Read the model definition and answer for the solid it produces. Units are mm, in the model's axes. Face numbers are marked on the shaded views. Coordinates: 2 decimals unless noted, no trailing zeros. Write each loop counter-clockwise with the first axis right and the second up, starting at its lowest first coordinate (ties: lowest second). Pieces come first, ordered by that corner, then holes. Notation, with made-up numbers: (-14.75, 50.5) -> (4.25, 50.5) arc R20 ccw to (4.25, 63.5) -> close; hole circle Ø10 at (-22.5, 23.25). An arc over 180 degrees is marked (long way). Answer as a JSON object with one key per item and string values. Group by question number.
(1) Find section B-B (x = -5.2). Give the vertices of the cut face in (y, z), then the cut area to 3 significant figures.
(2) Find section A-A (y = 18). Give the vertices of the cut face in (x, z).
(3) For a pull along X with two mould halves and no side action, classify the marked faces 1, 2, 3 and 4 as +X half, -X half, draft (parallel to the pull), parting line (faces both ways), or undercut.
(4) Find section C-C (z = 2.1). Give the vertices of the cut face in (x, y).
(5) Flat-ended cylindrical pins translate along their axes: P1, Ø1.5, axis at y = 8, z = 0.5, coming from the -X side; P2, Ø1.6, axis at x = 10, z = 1, coming from the +Y side; P3, Ø1.5, axis at y = 10.5, z = 2, coming from the +X side. Find the tip coordinate at first contact, or state that the pin passes through.
(6) Straight lines are drawn through the part: L1, parallel to Y at x = -3.5, z = 1.4; L2, parallel to Y at x = 0, z = 1; L3, parallel to X at y = 8, z = 1.55. For each, find the intervals that lie inside material, in ascending order.
(7) Find section D-D (x = 15). Give the vertices of the cut face in (y, z).
from build123d import *

# Parameters (mm, degrees)
SKETCH1_R           = 3.95
SKETCH1_R_2         = 1.5
BOSS_EXTRUDE1_DEPTH = 3
FILLET1_R           = 20
FILLET2_R           = 3
CUT_EXTRUDE1_DEPTH  = 3


with BuildPart() as part:
    # Sketch1 → Boss-Extrude1 (new body)
    with BuildSketch(Plane.XY):
        with BuildLine():
            Line((0, 41.674052381), (9.1, 41.674052381))
            Line((9.1, 41.674052381), (9.1, 35.674052381))
            Line((9.1, 35.674052381), (11.1, 35.674052381))
            Line((11.1, 35.674052381), (11.1, 41.674052381))
            Line((11.1, 41.674052381), (20.2, 41.674052381))
            Line((20.2, 41.674052381), (20.2, 31.674052381))
            Line((20.2, 31.674052381), (12, 31.674052381))
            Line((12, 31.674052381), (12, 0))
            ThreePointArc((12, 0), (0, -12), (-12, 0))
            Line((-12, 0), (-12, 31.674052381))
            Line((-12, 31.674052381), (-20.2, 31.674052381))
            Line((-20.2, 31.674052381), (-20.2, 41.674052381))
            Line((-20.2, 41.674052381), (-11.1, 41.674052381))
            Line((-11.1, 41.674052381), (-11.1, 35.674052381))
            Line((-11.1, 35.674052381), (-9.1, 35.674052381))
            Line((-9.1, 35.674052381), (-9.1, 41.674052381))
            Line((-9.1, 41.674052381), (0, 41.674052381))
        make_face()
        Circle(SKETCH1_R, mode=Mode.SUBTRACT)
        with Locations((-15, 37.024052381)):
            Circle(SKETCH1_R_2, mode=Mode.SUBTRACT)
        with Locations((-5.2, 37.024052381)):
            Circle(SKETCH1_R_2, mode=Mode.SUBTRACT)
        with Locations((5.2, 37.024052381)):
            Circle(SKETCH1_R_2, mode=Mode.SUBTRACT)
        with Locations((15, 37.024052381)):
            Circle(SKETCH1_R_2, mode=Mode.SUBTRACT)
    extrude(amount=BOSS_EXTRUDE1_DEPTH)

    # Fillet1
    # the kernel refuses this fillet: 20 mm, written as the material it adds along each edge
    with BuildSketch(Plane(origin=(-12, 31.674052381, 0), x_dir=(0, -1, 0), z_dir=(0, 0, 1))) as fillet1_piece_1:
        with BuildLine():
            CenterArc((16.1480649, -20), FILLET1_R, 90, 53.842991799)
            Line((0, -8.2), (-0.322961298, -7.964))
            ThreePointArc((-0.322961298, -7.964), (-0.4, -4.1), (-0.4, 0))
            Line((-0.4, 0), (0, 0.4))
            Line((0, 0.4), (16.1480649, 0.4))
            Line((16.1480649, 0.4), (16.1480649, 0))
        make_face()
    extrude(amount=3)
    with BuildSketch(Plane(origin=(12, 31.674052381, 0), x_dir=(0, -1, 0), z_dir=(0, 0, 1))) as fillet1_piece_2:
        with BuildLine():
            CenterArc((16.1480649, 20), FILLET1_R, 216.157008201, 53.842991799)
            Line((0, 8.2), (-0.322961298, 7.964))
            ThreePointArc((-0.322961298, 7.964), (-0.4, 4.1), (-0.4, 0))
            Line((-0.4, 0), (0, -0.4))
            Line((0, -0.4), (16.1480649, -0.4))
            Line((16.1480649, -0.4), (16.1480649, 0))
        make_face()
    extrude(amount=3)

    # Fillet2
    fillet2_edges = [part.edges().sort_by_distance(p)[0] for p in [
        (20.2, 31.674052381, 1.5),
        (-20.2, 31.674052381, 1.5),
    ]]
    fillet(fillet2_edges, radius=FILLET2_R)

    # Sketch2 → Cut-Extrude1 (cut)
    with BuildSketch(Plane.XY.offset(3)):
        with BuildLine():
            Line((-10.690189186, 25.65418917), (1.597091478, 17.050542625))
            ThreePointArc((1.597091478, 17.050542625), (3.686184199, 17.418906036), (3.317820787, 19.507998757))
            Line((3.317820787, 19.507998757), (-8.969459877, 28.111645303))
            ThreePointArc((-8.969459877, 28.111645303), (-11.058552598, 27.743281891), (-10.690189186, 25.65418917))
        make_face()
    extrude(amount=-CUT_EXTRUDE1_DEPTH, mode=Mode.SUBTRACT)


solid = part.part
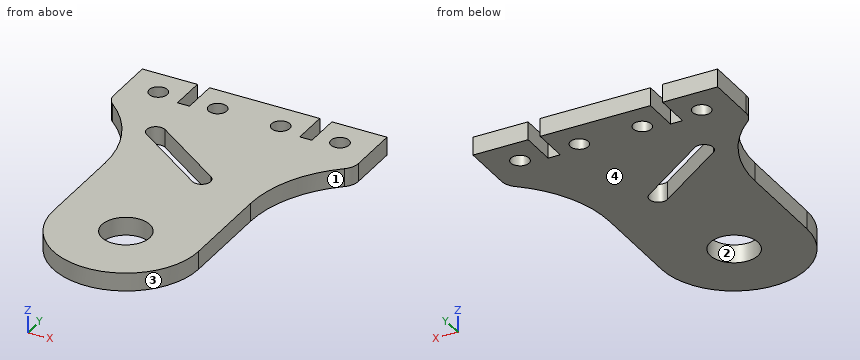
Results below:
{
 "1": {"outline": "(-10.81, 0) -> (21.81, 0) -> (21.81, 3) -> (-10.81, 3) -> close; (25.47, 0) -> (35.52, 0) -> (35.52, 3) -> (25.47, 3) -> close; (38.52, 0) -> (41.67, 0) -> (41.67, 3) -> (38.52, 3) -> close", "area": "137 mm2"},
 "2": {"outline": "(-12.15, 0) -> (0.24, 0) -> (0.24, 3) -> (-12.15, 3) -> close; (3.93, 0) -> (12.15, 0) -> (12.15, 3) -> (3.93, 3) -> close"},
 "3": {"face 1": "+X half", "face 2": "undercut", "face 3": "parting line", "face 4": "draft"},
 "4": {"outline": "(-20.2, 33.13) arc R3 ccw to (-19.13, 30.84) arc R20 cw to (-12, 15.53) -> (-12, 0) arc R12 ccw to (12, 0) -> (12, 15.53) arc R20 cw to (19.13, 30.84) arc R3 ccw to (20.2, 33.13) -> (20.2, 41.67) -> (11.1, 41.67) -> (11.1, 35.67) -> (9.1, 35.67) -> (9.1, 41.67) -> (-9.1, 41.67) -> (-9.1, 35.67) -> (-11.1, 35.67) -> (-11.1, 41.67) -> (-20.2, 41.67) -> close; hole circle Ø3 at (-15, 37.02); hole (-10.69, 25.65) -> (1.6, 17.05) arc R1.5 ccw to (3.32, 19.51) -> (-8.97, 28.11) arc R1.5 ccw to start; hole circle Ø3 at (-5.2, 37.02); hole circle Ø7.9 at (0, 0); hole circle Ø3 at (5.2, 37.02); hole circle Ø3 at (15, 37.02)"},
 "5": {"P1": "stops at x = -12", "P2": "stops at y = 35.67", "P3": "stops at x = 12"},
 "6": {"L1": "y = -11.48 to -1.83, 1.83 to 20.62, 24.28 to 41.67", "L2": "y = -12 to -3.95, 3.95 to 18.17, 21.83 to 41.67", "L3": "x = -12 to 12"},
 "7": {"outline": "(26.06, 0) -> (35.52, 0) -> (35.52, 3) -> (26.06, 3) -> close; (38.52, 0) -> (41.67, 0) -> (41.67, 3) -> (38.52, 3) -> close"}
}
